Autodesk Inventor part; units mm, degrees
ref_plane "YZ Plane" through (0, 0, 0) normal (1, 0, 0) x (0, 1, 0)
ref_plane "XZ Plane" through (0, 0, 0) normal (0, 1, 0) x (-1, 0, 0)
ref_plane "XY Plane" through (0, 0, 0) normal (0, 0, 1) x (1, 0, 0)
sketch "Esquisse1" plane through (0, 0, 0) normal (0, 0, 1) x (1, 0, 0)
  line L0 (0, 0) -> (34.4, 0)
  line L1 (34.4, 0) -> (34.4, 20)
  line L2 (34.4, 20) -> (0, 20)
  line L3 (0, 20) -> (0, 0)
  dimension "d0" = 34.4
  dimension "d1" = 20
extrude "Extrusion1" add sketch "Esquisse1" along normal blind 2.2
sketch "Esquisse2" plane through (0, 0, 2.2) normal (0, 0, 1) x (1, 0, 0)
  line L0 (0, 0) -> (34.4, 0)
  line L1 (34.4, 20) -> (0, 20)
  line L2 (0, 20) -> (0, 0)
  line L3 (0, 20) -> (2.2, 20)
  line L4 (2.2, 20) -> (2.2, 0)
  line L5 (2.2, 0) -> (0, 0)
  line L6 (0, 0) -> (0, 20)
  line L7 (17.2, 20) -> (17.2, 0) construction
  line L8 (34.4, 20) -> (32.2, 20)
  line L9 (32.2, 20) -> (32.2, 0)
  line L10 (32.2, 0) -> (34.4, 0)
  line L11 (34.4, 0) -> (34.4, 20)
  dimension "d4" = 2.2
extrude "Extrusion2" add sketch "Esquisse2" along normal blind 37 contours L2 L1 L4 L0 | L9 L1 L11 L0
sketch "Esquisse3" plane through (34.4, 0, 0) normal (1, 0, 0) x (0, 0, -1)
  line L0 (0, 0) -> (0, 20) construction
  line L1 (-39.2, 0) -> (-39.2, 20) construction
  line L2 (-39.2, 10) -> (0, 10) construction
  circle A0 centre (-30.2, 10) radius 2.15
  line L3 (-30.2, 10) -> (-30.2, 15.2246) construction
  circle A1 centre (-24.2, 10) radius 2.15
  circle A2 centre (-36.2, 10) radius 2.15
  circle A3 centre (-30.2, 10) radius 2.15
  circle A4 centre (-30.2, 16) radius 2.15
  circle A5 centre (-30.2, 4) radius 2.15
  circle A6 centre (-30.2, 10) radius 2.15
  dimension "d7" = 9
  dimension "d8" = 4.3
  dimension "d11" = 6
  dimension "d14" = 6
  dimension "d19" = 6
  dimension "d22" = 6
extrude "Extrusion3" cut sketch "Esquisse3" against normal through all
fillet "Congé1" radius 8 4 edges at (33.3, 20, 39.2) (1.1, 20, 39.2) (1.1, 0, 39.2) (33.3, 0, 39.2)
fillet "Congé2" radius 8 4 edges at (2.2, 10, 2.2) (0, 10, 0) (34.4, 10, 0) (32.2, 10, 2.2)
equation "\"d2\" = UDepth"
equation "\"d4\" = Depth"
equation "\"d8\" = Holes"
equation "\"d28\" = URound"
equation "\"Depth\" = 2.2"
equation "\"Holes\" = 4.3"
equation "\"UDepth\" = Depth"
equation "\"USize\" = 5"
equation "\"URound\" = 8"
properties part number "BackFeet"
For this review, take the finished solid that the model builds, in its own axes (mm). A direction names the side the tool comes from. Coordinates: 2 decimals unless noted, no trailing zeros. Write each loop counter-clockwise with the first axis right and the second up, starting at its lowest first coordinate (ties: lowest second). Pieces come first, ordered by that corner, then holes. Notation, with made-up numbers: (39, 35.5) - (56, 35.5) arc R28 cw to (56, 59.5) - close; hole circle Ø2 at (-25.75, 82.25). An arc over 180 degrees is marked (long way). Answer in a Markdown table with one row per item. Add a question column.
Q1. We need section B-B, the plane z = 24.2. State the section outline as (x, y) points, and give its area (3 significant figures).
Q2. Tool access review of faces 4 (the flat face through (17, 10, 2.2)), 5 (the cylindrical face through (33.32, 10.65, 34.15)): name each direction out of +Z, -Z, +X, -X, +Y, -Y from which nothing blocks a thin tool from reaching the whole face with its end or side.
Q3. Draft analysis for pull direction Z (two halves, no side actions). For faces 1 (the cylindrical face through (33.315, 2.406, 36.919)), 2 (the cylindrical face through (1.12, 10.65, 28.15)), 3 (the flat face through (17, 10, 0)), state which applies: +Z half, -Z half, draft (parallel to the pull), parting line (faces both ways), or undercut.
Q4. We need section C-C, the plane z = 30.2. Count the separate pieces of the cut face and the enclosed holes in it, and give its area (3 significant figures).
Q5. We need section A-A, the plane z = 17. State the section outline as (x, y) points.
Q6. For probe 1 along Y at (x, z) = (0.8, 30.2); probe 2 along X at (y, z) = (17, 24.5); probe 3 along Z at (x, y) = (20.5, 2.75), list the stretches that pass through material, from the lowest coordinate up.
Q7. For P1, Ø5, axis at x = 6.5, y = 10, coming from the +Z side; P2, Ø4, axis at x = 27.5, y = 15.5, coming from the +Z side; P3, Ø1.5, axis at x = 9.5, y = 5.5, coming from the +Z side, all flat-tipped, find the tip position at first contact; note any pin that passes through.
Answer list:
| question | item | result |
|---|---|---|
| 1 | outline | (0, 0) - (2.2, 0) - (2.2, 7.85) - (0, 7.85) - close; (0, 12.15) - (2.2, 12.15) - (2.2, 20) - (0, 20) - close; (32.2, 0) - (34.4, 0) - (34.4, 7.85) - (32.2, 7.85) - close; (32.2, 12.15) - (34.4, 12.15) - (34.4, 20) - (32.2, 20) - close |
| 1 | area | 69.1 mm2 |
| 2 | face 4 | +Z, +Y, -Y |
| 2 | face 5 | +X, -X |
| 3 | face 1 | +Z half |
| 3 | face 2 | undercut |
| 3 | face 3 | -Z half |
| 4 | separate pieces | 8 |
| 4 | enclosed holes | 0 |
| 4 | area | 31.2 mm2 |
| 5 | outline | (0, 0) - (2.2, 0) - (2.2, 20) - (0, 20) - close; (32.2, 0) - (34.4, 0) - (34.4, 20) - (32.2, 20) - close |
| 6 | probe 1 | y = 0 to 1.85, 6.15 to 7.85, 12.15 to 13.85, 18.15 to 20 |
| 6 | probe 2 | x = 0 to 2.2, 32.2 to 34.4 |
| 6 | probe 3 | z = 0 to 2.2 |
| 7 | P1 | stops at z = 5.14 |
| 7 | P2 | stops at z = 4.21 |
| 7 | P3 | stops at z = 2.33 |
